Drawing for the job (mm, zero at the part's lowest x, y, z). A direction names the side the tool comes from. Coordinates: 2 decimals unless noted, no trailing zeros. Loops run counter-clockwise (first coordinate to the right, second up) from the corner with the lowest first, then second, coordinate; pieces in that order, holes last. Notation, with made-up numbers: (-2.75, 58.25) -> (19.25, 58.25) arc R4 cw to (19.25, 64.25) -> close; hole circle Ø8 at (17, 10.5). An arc over 180 degrees is marked (long way). Write each question's results on one line, items separated by ' | '.
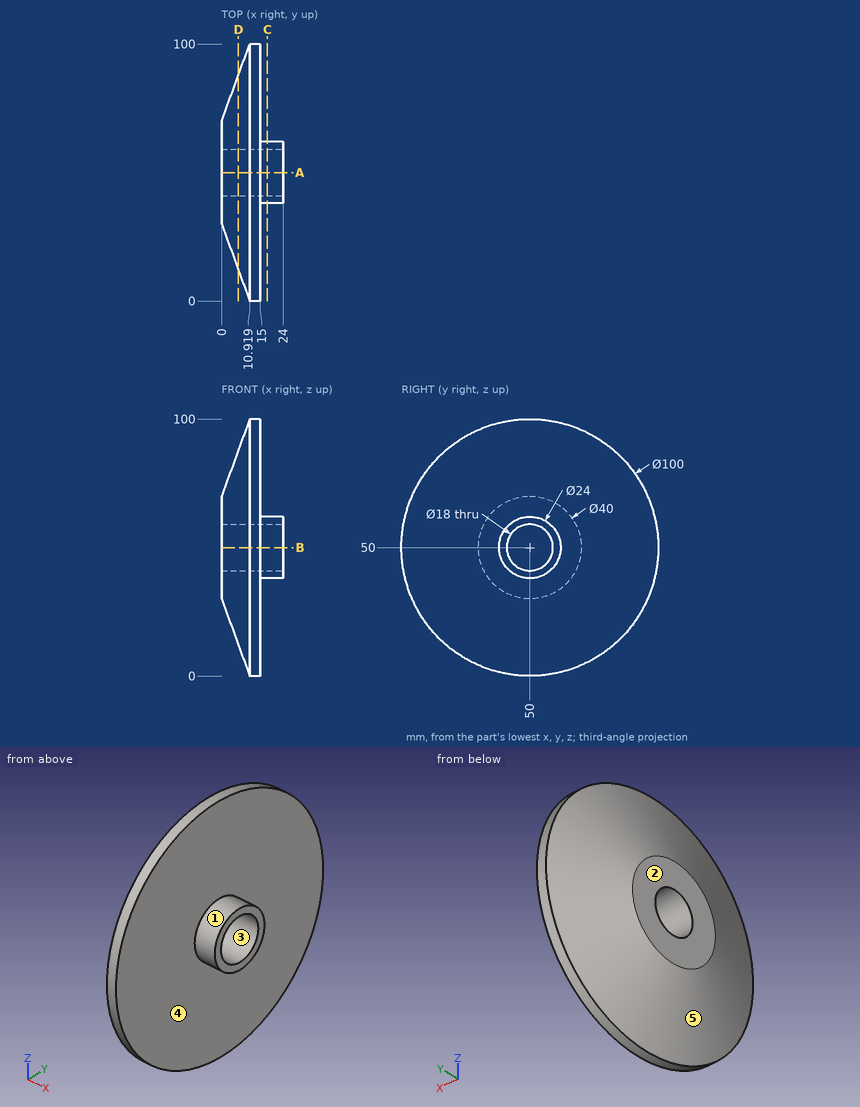
1) Two-plate mould, pull along Y, no slides. Class the marked faces 1, 2 and 3: pulls with the +Y half, pulls with the -Y half, needs draft (parallel to the pull), parting line crosses it, or undercut.
Outcome:
face 1: parting line crosses it | face 2: needs draft | face 3: undercut
2) Slice it at D-D (x = 6.5). Write the cut outline in (y, z), then the cut area to 3 significant figures.
Outcome:
outline: circle Ø75.72 at (50, 50); hole circle Ø18 at (50, 50) | area: 4,250 mm^2
3) Which spindle directions (+Z, -Z, +X, -X, +Y, -Y) get a long thin tool onto all of the face, cutting with end or side? Do the marked faces 4 and 5. Say none if no direction does.
Outcome:
face 4: +X | face 5: -X
4) Slice it at A-A (y = 50). Write the cut outline in (x, z), then the cut area to 3 significant figures.
Outcome:
outline: (0, 30) -> (10.92, 0) -> (15, 0) -> (15, 38) -> (24, 38) -> (24, 41) -> (0, 41) -> close; (0, 59) -> (24, 59) -> (24, 62) -> (15, 62) -> (15, 100) -> (10.92, 100) -> (0, 70) -> close | area: 956 mm^2
5) Slice it at C-C (x = 17.75). Write the cut outline in (y, z).
Outcome:
outline: circle Ø24 at (50, 50); hole circle Ø18 at (50, 50)
6) Drill centre lines: L1, parallel to Y at x = 18.5, z = 48 (3 decimals); L2, parallel to Y at x = 21.25, z = 58 (1 decimal); L3, parallel to X at y = 46, z = 32.5. Where is each one in solid material? Low to high. Write a range as from..to.
Outcome:
L1: y = 38.168..41.225, 58.775..61.832 | L2: y = 41.1..45.9, 54.1..58.9 | L3: x = 0..15
7) Pin check, flat tips, straight feed: pin 1 (5 mm diameter, centred on x = 18.5, z = 71.5, fed in from +Y); pin 2 (2 mm diameter, centred on y = 21, z = 11.5, fed in from -X); pin 3 (5 mm diameter, centred on y = 53.5, z = 24, fed in from -X); pin 4 (1.5 mm diameter, centred on y = 31, z = 30, fed in from -X). Stop position of each tip, or through.
Outcome:
pin 1: passes through | pin 2: stops at x = 9.9 | pin 3: stops at x = 1.36 | pin 4: stops at x = 2.49
